```python
from build123d import *

# Parameters (mm, degrees)
BOSS_EXTRUDE1_DEPTH = 36.5
BOSS_EXTRUDE2_DEPTH = 6
BOSS_EXTRUDE3_DEPTH = 15
BOSS_EXTRUDE4_DEPTH = 18
CUT_EXTRUDE2_DEPTH  = 25
SKETCH5_W           = 21
SKETCH5_H           = 37.8
CUT_EXTRUDE1_DEPTH  = 32
FILLET1_R           = 10
CUT_EXTRUDE3_DEPTH  = 18
SKETCH9_W           = 86.823098523
SKETCH9_H           = 11.225168108
CUT_EXTRUDE4_DEPTH  = 18


with BuildPart() as part:
    # Sketch1 → Boss-Extrude1 (new body)
    with BuildSketch(Plane(origin=(0, 0, 0), x_dir=(1, 0, 0), z_dir=(0, 1, 0))):
        with BuildLine():
            Line((-62.5, -34.2), (-62.5, -35.745629103))
            ThreePointArc((-62.5, -35.745629103), (0, -72), (62.5, -35.745629103))
            Line((62.5, -35.745629103), (62.5, -34.2))
            Line((62.5, -34.2), (-62.5, -34.2))
        make_face()
    extrude(amount=-BOSS_EXTRUDE1_DEPTH)

    # Sketch2 → Boss-Extrude2 (add)
    with BuildSketch(Plane.XZ.offset(36.5)):
        with BuildLine():
            ThreePointArc((39.5, 60.197591314), (0, 72), (-39.5, 60.197591314))
            Line((-39.5, 60.197591314), (-39.5, 34.2))
            Line((-39.5, 34.2), (39.5, 34.2))
            Line((39.5, 34.2), (39.5, 60.197591314))
        make_face()
    extrude(amount=BOSS_EXTRUDE2_DEPTH)

    # Sketch3 → Boss-Extrude3 (add)
    with BuildSketch(Plane.XZ.offset(42.5)):
        with BuildLine():
            Line((-32, 64.498061986), (-32, 34.2))
            Line((-32, 34.2), (32, 34.2))
            Line((32, 34.2), (32, 64.498061986))
            ThreePointArc((32, 64.498061986), (0, 72), (-32, 64.498061986))
        make_face()
    extrude(amount=BOSS_EXTRUDE3_DEPTH)

    # Sketch4 → Boss-Extrude4 (add)
    with BuildSketch(Plane.XZ.offset(57.5)):
        with BuildLine():
            Line((-24.5, 34.2), (-24.5, 67.703397256))
            ThreePointArc((-24.5, 67.703397256), (0, 72), (24.5, 67.703397256))
            Line((24.5, 67.703397256), (24.5, 34.2))
            Line((24.5, 34.2), (-24.5, 34.2))
        make_face()
    extrude(amount=BOSS_EXTRUDE4_DEPTH)

    # Sketch7 → Cut-Extrude2 (cut)
    with BuildSketch(Plane(origin=(0, 0, 34.2), x_dir=(-1, 0, 0), z_dir=(0, 0, -1))):
        with BuildLine():
            Line((-32.5, -53.5), (-32.5, -86))
            Line((-32.5, -86), (32.5, -86))
            Line((32.5, -86), (32.5, -53.5))
            ThreePointArc((32.5, -53.5), (0, -21), (-32.5, -53.5))
        make_face()
    extrude(amount=-CUT_EXTRUDE2_DEPTH, mode=Mode.SUBTRACT)

    # Sketch5 → Cut-Extrude1 (cut)
    with BuildSketch(Plane.XZ.offset(75.5)):
        with Locations((0, 53.1)):
            Rectangle(SKETCH5_W, SKETCH5_H)
    extrude(amount=-CUT_EXTRUDE1_DEPTH, mode=Mode.SUBTRACT)

    # Fillet1
    fillet1_edges = [part.edges().sort_by_distance(p)[0] for p in [
        (-10.5, -43.5, 65.215130212),
        (10.5, -43.5, 65.215130212),
    ]]
    fillet(fillet1_edges, radius=FILLET1_R)

    # Sketch8 → Cut-Extrude3 (cut)
    with BuildSketch(Plane(origin=(0, 0, 34.2), x_dir=(-1, 0, 0), z_dir=(0, 0, -1))):
        with BuildLine():
            Line((-27, 0), (27, 0))
            ThreePointArc((27, 0), (49, -22), (27, -44))
            Line((27, -44), (-27, -44))
            ThreePointArc((-27, -44), (-49, -22), (-27, 0))
        make_face()
    extrude(amount=-CUT_EXTRUDE3_DEPTH, mode=Mode.SUBTRACT)

    # Sketch9 → Cut-Extrude4 (cut)
    with BuildSketch(Plane(origin=(0, 0, 34.2), x_dir=(-1, 0, 0), z_dir=(0, 0, -1))):
        with Locations((0.144250153, -44.182683468)):
            Rectangle(SKETCH9_W, SKETCH9_H)
    extrude(amount=-CUT_EXTRUDE4_DEPTH, mode=Mode.SUBTRACT)


solid = part.part
```
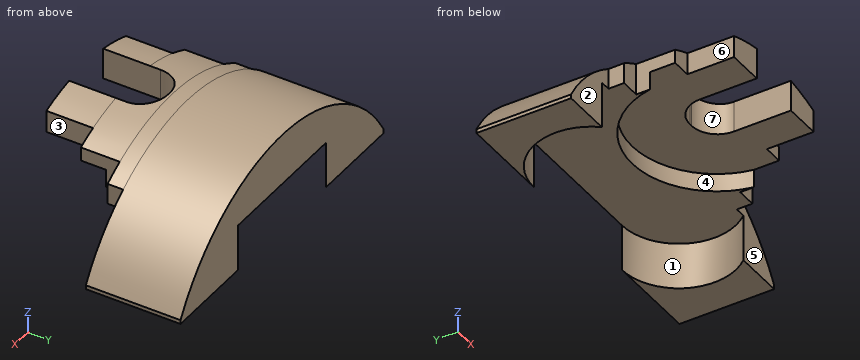
For this review, take the finished solid that the model builds, in its own axes (mm). Face numbers are marked on the shaded views. A direction names the side the tool comes from. Coordinates: 2 decimals unless noted, no trailing zeros. Loops run counter-clockwise (first coordinate to the right, second up) from the corner with the lowest first, then second, coordinate; pieces in that order, holes last. Notation, with made-up numbers: (60, -21) - (119, -21) arc R27 ccw to (119, 3) - close; hole circle Ø6 at (-0.5, -40). An arc over 180 degrees is marked (long way). Use one line per item in the form item = value. Start each with the question number.
1) Draft analysis for pull direction X (two halves, no side actions). For the marked faces 1, 2 and 3, state which applies: released by +X, released by -X, zero draft, split by the parting line, or undercut.
2) Take a section at D-D (z = 55.5). State the section outline as (x, y) points.
3) For pin 1 (5 mm diameter, centred on y = -38.5, z = 57, fed in from +X); pin 2 (14.5 mm diameter, centred on x = -22.5, y = -16.5, fed in from -Z); pin 3 (0.5 mm diameter, centred on x = 0, z = 66.5, fed in from -Y); pin 4 (1.5 mm diameter, centred on x = -37, z = 40.5, fed in from +Y), all flat-tipped, find the tip position at first contact; note any pin that passes through.
4) To check wall thickness, follow probe 1 along Y at (x, z) = (-1, 66); probe 2 along X at (y, z) = (-40.5, 54.5); probe 3 along X at (y, z) = (-25, 43). State the ranges of each line that lie inside material, in increasing order. Write a range as from..to.
5) Take a section at A-A (y = -45.5). State the section outline as (x, z) points.
6) Take a section at B-B (z = 37.5). State the section outline as (x, y) points.
7) For the marked faces 4, 5, 6 and 7, list the 3-axis set-ups (+Z, -Z, +X, -X, +Y, -Y) from which the entire face can be reached by the end or side of a thin tool; tool diameter is ignored.
8) Take a section at C-C (x = 20.5). State the section outline as (y, z) points, plus the area to 3 significant figures.
From the geometry:
q1.face_1 = undercut
q1.face_2 = zero draft
q1.face_3 = released by +X
q2.outline = (-45.87, -36.5) - (-39.5, -36.5) - (-39.5, -42.5) - (-32, -42.5) - (-32, -47.82) arc R32.5 cw to (32, -47.82) - (32, -42.5) - (39.5, -42.5) - (39.5, -36.5) - (45.87, -36.5) - (45.87, 0) - (-45.87, 0) - close
q3.pin_1 = 45.87
q3.pin_2 = 52.2
q3.pin_3 = -43.5
q3.pin_4 = 0
q4.probe_1 = -43.51..0
q4.probe_2 = -39.5..-29.79, 29.79..39.5
q4.probe_3 = -57.75..-48.79, 48.79..57.75
q5.outline = (-32, 52.2) - (-31.5, 52.2) - (-31.5, 59.2) - (-6.5, 59.2) - (-6.5, 71.71) arc R72 ccw to (-32, 64.5) - close; (6.5, 59.2) - (31.5, 59.2) - (31.5, 52.2) - (32, 52.2) - (32, 64.5) arc R72 ccw to (6.5, 71.71) - close
q6.outline = (-61.46, -36.5) - (-43.55, -36.5) arc R22 cw to (-27, 0) - (-61.46, 0) - close; (27, 0) arc R22 cw to (43.55, -36.5) - (61.46, -36.5) - (61.46, 0) - close
q7.face_4 = -Z, -Y
q7.face_5 = +Z, -Z, +X, -Y
q7.face_6 = +Z, -Z, -X, -Y
q7.face_7 = +Z, -Z, -Y
q8.outline = (-75.5, 59.2) - (-28.28, 59.2) - (-28.28, 52.2) - (0, 52.2) - (0, 69.02) - (-75.5, 69.02) - close
q8.area = 939 mm2
